Autodesk Inventor part; units mm, degrees
ref_plane "YZ Plane" through (0, 0, 0) normal (1, 0, 0) x (0, 1, 0)
ref_plane "XZ Plane" through (0, 0, 0) normal (0, 1, 0) x (-1, 0, 0)
ref_plane "XY Plane" through (0, 0, 0) normal (0, 0, 1) x (1, 0, 0)
sketch "Sketch1" plane through (0, 0, 0) normal (0, 1, 0) x (-1, 0, 0)
  circle A0 centre (0, 0) radius 2.5
  circle A1 centre (0, 0) radius 1
  dimension "d0" = 5
extrude "Extrusion1" add sketch "Sketch1" against normal blind 10 contours A1
sketch "Sketch2" plane through (0, 0, 0) normal (0, 1, 0) x (1, 0, 0)
  circle A0 centre (0, 0) radius 2
  dimension "d3" = 4
extrude "Extrusion2" add sketch "Sketch2" along normal blind 2
sketch "Sketch3" plane through (0, 2, 0) normal (0, 1, 0) x (1, 0, 0)
  circle A0 centre (0, 0) radius 1
  line L0 (0, 1) -> (0.866, 0.5)
  line L1 (0.866, 0.5) -> (0.866, -0.5)
  line L2 (0.866, -0.5) -> (0, -1)
  line L3 (0, -1) -> (-0.866, -0.5)
  line L4 (-0.866, -0.5) -> (-0.866, 0.5)
  line L5 (-0.866, 0.5) -> (0, 1)
extrude "Extrusion3" cut sketch "Sketch3" against normal blind 0.5 contours L1 L2 L3 L4 L5 L0
properties part number "4mm_screw" material "Stainless Steel"
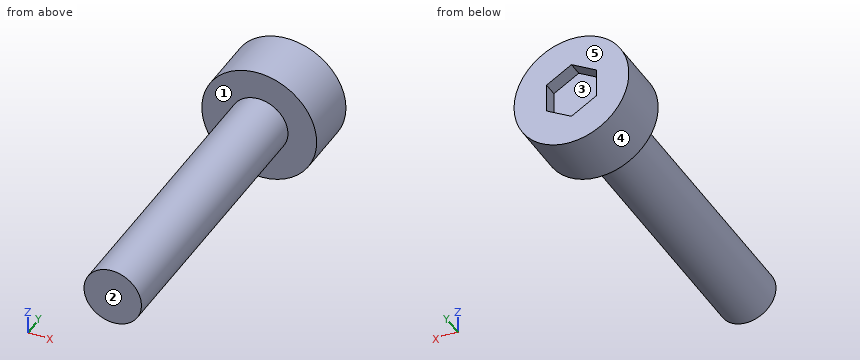
Design review of the part built by this model. Coordinates are the model's own, in mm. Face numbers are marked on the shaded views. A direction names the side the tool comes from. Coordinates: 2 decimals unless noted, no trailing zeros. Write each loop counter-clockwise with the first axis right and the second up, starting at its lowest first coordinate (ties: lowest second). Pieces come first, ordered by that corner, then holes.
1) Add section D-D (x = -1.2). Write out the cut boundary in (y, z).
2) Mouldability with a two-part tool opening along X and no side actions: class the marked faces 3, 4 and 5 as +X half, -X half, draft (parallel to the pull), parting line (faces both ways), or undercut.
3) Add section B-B (x = 0.7). Write out the cut boundary in (y, z).
4) To check wall thickness, follow L1, parallel to Y at x = -1.4, z = 0; L2, parallel to Z at x = 0.1, y = 1.75; L3, parallel to Y at x = 0.5, z = -0.45. State the ranges of each line that lie inside material, in increasing order.
5) Add section A-A (z = 0). Write out the cut boundary in (x, y), plus the area to 3 significant figures.
6) Add section C-C (y = -4). Write out the cut boundary in (x, z).
7) Machinability: for the marked faces 1 and 2, which of the approach directions +Z, -Z, +X, -X, +Y, -Y give a long, thin tool a straight path to every point of the face, cutting with its end or side? Answer none if there is none.
8) Insertion check: pin 1 (2 mm diameter, centred on x = -1.5, y = -1.5, fed in from +Z); pin 2 (2 mm diameter, centred on y = -4, z = -0.5, fed in from -X). Each pin has a flat end and moves straight along its axis. Give the tip position at first contact, or say it passes through.
Check result:
1. outline: (0, -1.6) - (2, -1.6) - (2, 1.6) - (0, 1.6) - close
2. face 3: undercut
2. face 4: parting line
2. face 5: draft
3. outline: (-10, -0.71) - (0, -0.71) - (0, -1.87) - (2, -1.87) - (2, -0.6) - (1.5, -0.6) - (1.5, 0.6) - (2, 0.6) - (2, 1.87) - (0, 1.87) - (0, 0.71) - (-10, 0.71) - close
4. L1: y = 0 to 2
4. L2: z = -2 to -0.94, 0.94 to 2
4. L3: y = -10 to 1.5
5. outline: (-2, 0) - (-1, 0) - (-1, -10) - (1, -10) - (1, 0) - (2, 0) - (2, 2) - (0.87, 2) - (0.87, 1.5) - (-0.87, 1.5) - (-0.87, 2) - (-2, 2) - close
5. area: 27.1 mm2
6. outline: circle Ø2 at (0, 0)
7. face 1: -Y
7. face 2: +Z, -Z, +X, -X, -Y
8. pin 1: stops at z = 0.87
8. pin 2: stops at x = -1
